Verification items for the finished model (mm, model axes). Face numbers are marked on the shaded views. A direction names the side the tool comes from. Round coordinates to 2 decimals unless told otherwise and drop trailing zeros. Loops run counter-clockwise (first coordinate to the right, second up) from the corner with the lowest first, then second, coordinate; pieces in that order, holes last. Notation, with made-up numbers: (52, 2.25) -> (78, 2.25) arc R30 ccw to (78, 30.25) -> close; hole circle Ø4 at (-28.75, 60.25). An arc over 180 degrees is marked (long way). Write item = value, one per line.
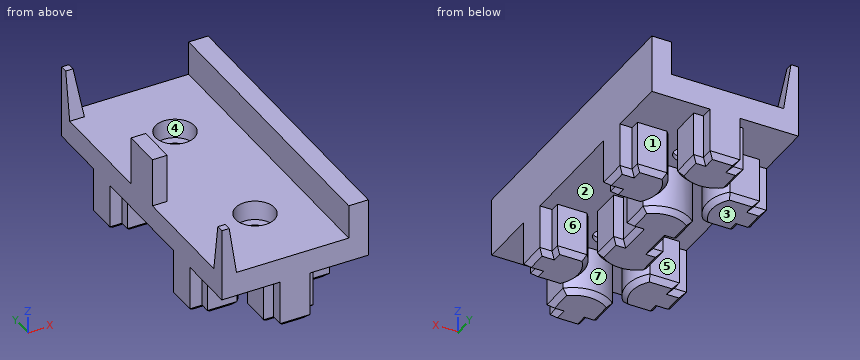
```python
from build123d import *

# Parameters (mm, degrees)
SKETCH_1_W                   = 30
SKETCH_1_H                   = 60
EXTRUDE_1_DEPTH              = 5
SKETCH_2_W                   = 3
SKETCH_2_H                   = 3
SKETCH_2_W_2                 = 4
SKETCH_2_H_2                 = 60
SKETCH_2_H_3                 = 8
EXTRUDE_2_DEPTH              = 10
CUT_EXTRUDE_1_DEPTH          = 44.058100283
CUT_EXTRUDE_3_DEPTH          = 7
SKETCH_5_W                   = 4
SKETCH_5_H                   = 3
CUT_EXTRUDE_4_DEPTH          = 64.639610307
HOLE_WIZARD_M4_1_D           = 4.5
HOLE_WIZARD_M4_1_CBORE_D     = 8
HOLE_WIZARD_M4_1_CBORE_DEPTH = 4
EXTRUDE_3_DEPTH              = 10
CHAMFER_1_SIZE               = 1


with BuildPart() as part:
    # 스케치1 → 보스-돌출1 (new body)
    with BuildSketch(Plane.XY):
        Rectangle(SKETCH_1_W, SKETCH_1_H)
    extrude(amount=EXTRUDE_1_DEPTH)

    # 스케치2 → 보스-돌출2 (add)
    with BuildSketch(Plane.XY.offset(5)):
        with Locations((-13.5, -28.5)):
            Rectangle(SKETCH_2_W, SKETCH_2_H)
        with Locations((-13.5, 28.5)):
            Rectangle(SKETCH_2_W, SKETCH_2_H)
        with Locations((13, 0)):
            Rectangle(SKETCH_2_W_2, SKETCH_2_H_2)
        with Locations((-13.5, 0)):
            Rectangle(SKETCH_2_W, SKETCH_2_H_3)
    extrude(amount=EXTRUDE_2_DEPTH)

    # 스케치3 → 컷-돌출1 (cut, through all)
    with BuildSketch(Plane(origin=(-12, 0, 0), x_dir=(0, 0, -1), z_dir=(1, 0, 0))):
        Polygon((-15, -28.5), (-5, -27), (-15, -27), align=None)
    cut_extrude_1 = extrude(amount=-CUT_EXTRUDE_1_DEPTH, mode=Mode.SUBTRACT)

    # 스케치4 → 컷-돌출3 (cut)
    with BuildSketch(Plane.XZ.offset(30)):
        Polygon((-13.5, 15), (-12, 15), (-12, 5), align=None)
    cut_extrude_3 = extrude(amount=-CUT_EXTRUDE_3_DEPTH, mode=Mode.SUBTRACT)

    # 대칭 복사1: 컷-돌출1, 컷-돌출3 across plane
    add(cut_extrude_1.mirror(Plane(origin=(0, 0, 0), x_dir=(0, 0, 1), z_dir=(0, -1, 0))), mode=Mode.SUBTRACT)
    add(cut_extrude_3.mirror(Plane(origin=(0, 0, 0), x_dir=(0, 0, 1), z_dir=(0, -1, 0))), mode=Mode.SUBTRACT)

    # 스케치5 → 컷-돌출4 (cut, through all)
    with BuildSketch(Plane(origin=(0, 30, 0), x_dir=(1, 0, 0), z_dir=(0, 1, 0))):
        with Locations((13, -13.5)):
            Rectangle(SKETCH_5_W, SKETCH_5_H)
    extrude(amount=-CUT_EXTRUDE_4_DEPTH, mode=Mode.SUBTRACT)

    # M4 소켓 머리 캡 나사용 카운터보어1 (through all)
    with Locations(Plane.XY.offset(5)):
        with Locations((0, -15), (0, 15)):
            CounterBoreHole(HOLE_WIZARD_M4_1_D / 2, HOLE_WIZARD_M4_1_CBORE_D / 2, HOLE_WIZARD_M4_1_CBORE_DEPTH)

    # 스케치9 → 보스-돌출3 (add)
    with BuildSketch(Plane(origin=(0, 0, 0), x_dir=(-1, 0, 0), z_dir=(0, 0, -1))):
        with BuildLine():
            Line((-3.05, 30), (3.05, 30))
            Line((3.05, 30), (3.05, 27.5))
            Line((3.05, 27.5), (5.05, 27.5))
            Line((5.05, 27.5), (5.05, 21.454957169))
            ThreePointArc((5.05, 21.454957169), (0, 19.5), (-5.05, 21.454957169))
            Line((-5.05, 21.454957169), (-5.05, 27.5))
            Line((-5.05, 27.5), (-3.05, 27.5))
            Line((-3.05, 27.5), (-3.05, 30))
        make_face()
        with BuildLine():
            Line((15, 18.05), (15, 11.95))
            Line((15, 11.95), (12.5, 11.95))
            Line((12.5, 11.95), (12.5, 9.95))
            Line((12.5, 9.95), (6.454957169, 9.95))
            ThreePointArc((6.454957169, 9.95), (4.5, 15), (6.454957169, 20.05))
            Line((6.454957169, 20.05), (12.5, 20.05))
            Line((12.5, 20.05), (12.5, 18.05))
            Line((12.5, 18.05), (15, 18.05))
        make_face()
        with BuildLine():
            Line((-3.05, 2.5), (-5.05, 2.5))
            Line((-5.05, 2.5), (-5.05, 8.545042831))
            ThreePointArc((-5.05, 8.545042831), (0, 10.5), (5.05, 8.545042831))
            Line((5.05, 8.545042831), (5.05, 2.5))
            Line((5.05, 2.5), (3.05, 2.5))
            Line((3.05, 2.5), (3.05, -2.5))
            Line((3.05, -2.5), (5.05, -2.5))
            Line((5.05, -2.5), (5.05, -8.545042831))
            ThreePointArc((5.05, -8.545042831), (0, -10.5), (-5.05, -8.545042831))
            Line((-5.05, -8.545042831), (-5.05, -2.5))
            Line((-5.05, -2.5), (-3.05, -2.5))
            Line((-3.05, -2.5), (-3.05, 2.5))
        make_face()
        with BuildLine():
            Line((-15, 11.95), (-15, 18.05))
            Line((-15, 18.05), (-12.5, 18.05))
            Line((-12.5, 18.05), (-12.5, 20.05))
            Line((-12.5, 20.05), (-6.454957169, 20.05))
            ThreePointArc((-6.454957169, 20.05), (-4.5, 15), (-6.454957169, 9.95))
            Line((-6.454957169, 9.95), (-12.5, 9.95))
            Line((-12.5, 9.95), (-12.5, 11.95))
            Line((-12.5, 11.95), (-15, 11.95))
        make_face()
        with BuildLine():
            Line((-5.05, -27.5), (-5.05, -21.454957169))
            ThreePointArc((-5.05, -21.454957169), (0, -19.5), (5.05, -21.454957169))
            Line((5.05, -21.454957169), (5.05, -27.5))
            Line((5.05, -27.5), (3.05, -27.5))
            Line((3.05, -27.5), (3.05, -30))
            Line((3.05, -30), (-3.05, -30))
            Line((-3.05, -30), (-3.05, -27.5))
            Line((-3.05, -27.5), (-5.05, -27.5))
        make_face()
        with BuildLine():
            Line((-12.5, -9.95), (-6.454957169, -9.95))
            ThreePointArc((-6.454957169, -9.95), (-4.5, -15), (-6.454957169, -20.05))
            Line((-6.454957169, -20.05), (-12.5, -20.05))
            Line((-12.5, -20.05), (-12.5, -18.05))
            Line((-12.5, -18.05), (-15, -18.05))
            Line((-15, -18.05), (-15, -11.95))
            Line((-15, -11.95), (-12.5, -11.95))
            Line((-12.5, -11.95), (-12.5, -9.95))
        make_face()
        with BuildLine():
            Line((12.5, -20.05), (6.454957169, -20.05))
            ThreePointArc((6.454957169, -20.05), (4.5, -15), (6.454957169, -9.95))
            Line((6.454957169, -9.95), (12.5, -9.95))
            Line((12.5, -9.95), (12.5, -11.95))
            Line((12.5, -11.95), (15, -11.95))
            Line((15, -11.95), (15, -18.05))
            Line((15, -18.05), (12.5, -18.05))
            Line((12.5, -18.05), (12.5, -20.05))
        make_face()
    extrude(amount=EXTRUDE_3_DEPTH)

    # 모따기1
    chamfer_1_edges = [part.edges().sort_by_distance(p)[0] for p in [
        (3.05, 28.75, -10),
        (4.05, 27.5, -10),
        (5.05, 24.477478584, -10),
        (0, 19.5, -10),
        (-5.05, 24.477478584, -10),
        (-4.05, 27.5, -10),
        (-3.05, 28.75, -10),
        (0, 30, -10),
        (-13.75, 18.05, -10),
        (-12.5, 19.05, -10),
        (-9.477478584, 20.05, -10),
        (-4.5, 15, -10),
        (-9.477478584, 9.95, -10),
        (-12.5, 10.95, -10),
        (-13.75, 11.95, -10),
        (-15, 15, -10),
        (3.05, 0, -10),
        (4.05, -2.5, -10),
        (5.05, -5.522521416, -10),
        (0, -10.5, -10),
        (-5.05, -5.522521416, -10),
        (-4.05, -2.5, -10),
        (-3.05, 0, -10),
        (-4.05, 2.5, -10),
        (-5.05, 5.522521416, -10),
        (0, 10.5, -10),
        (5.05, 5.522521416, -10),
        (4.05, 2.5, -10),
        (13.75, 11.95, -10),
        (12.5, 10.95, -10),
        (9.477478584, 9.95, -10),
        (4.5, 15, -10),
        (9.477478584, 20.05, -10),
        (12.5, 19.05, -10),
        (13.75, 18.05, -10),
        (15, 15, -10),
        (0, -19.5, -10),
        (5.05, -24.477478584, -10),
        (4.05, -27.5, -10),
        (3.05, -28.75, -10),
        (0, -30, -10),
        (-3.05, -28.75, -10),
        (-4.05, -27.5, -10),
        (-5.05, -24.477478584, -10),
        (4.5, -15, -10),
        (9.477478584, -9.95, -10),
        (12.5, -10.95, -10),
        (13.75, -11.95, -10),
        (15, -15, -10),
        (13.75, -18.05, -10),
        (12.5, -19.05, -10),
        (9.477478584, -20.05, -10),
        (-4.5, -15, -10),
        (-9.477478584, -20.05, -10),
        (-12.5, -19.05, -10),
        (-13.75, -18.05, -10),
        (-15, -15, -10),
        (-13.75, -11.95, -10),
        (-12.5, -10.95, -10),
        (-9.477478584, -9.95, -10),
    ]]
    chamfer(chamfer_1_edges, length=CHAMFER_1_SIZE)


solid = part.part
```
(1) Sectioned sample at B-B, the plane z = 8. Record the cut outline in (x, y), and give its area (3 significant figures).
Filled sheet:
outline = (-15, -30) -> (-12.45, -30) -> (-12.45, -27.45) -> (-15, -27.45) -> close; (-15, -4) -> (-12, -4) -> (-12, 4) -> (-15, 4) -> close; (-15, 27.45) -> (-12.45, 27.45) -> (-12.45, 30) -> (-15, 30) -> close; (11, -30) -> (15, -30) -> (15, 30) -> (11, 30) -> close
area = 277 mm2
(2) Go/stop test with flat-tipped pins: pin 1 Ø0.8 at (x, z) = (14, -4.5) entering from +Y; pin 2 Ø0.6 at (y, z) = (-18.5, -6) entering from -X; pin 3 Ø2 at (y, z) = (-28, -5.5) entering from -X; pin 4 Ø8 at (x, z) = (-5, -6) entering from +Y. Record where each tip stops, or that it passes through.
Filled sheet:
pin_1 = 18.05
pin_2 = -12.5
pin_3 = -5.05
pin_4 = 30
(3) Sectioned sample at A-A, the plane y = 15. Record the cut outline in (x, z), and give its area (4 significant figures).
Filled sheet:
outline = (-15, -9) -> (-14, -10) -> (-5.5, -10) -> (-4.5, -9) -> (-4.5, 0) -> (-2.25, 0) -> (-2.25, 1) -> (-4, 1) -> (-4, 5) -> (-15, 5) -> close; (2.25, 0) -> (4.5, 0) -> (4.5, -9) -> (5.5, -10) -> (14, -10) -> (15, -9) -> (15, 12) -> (11, 12) -> (11, 5) -> (4, 5) -> (4, 1) -> (2.25, 1) -> close
area = 349.5 mm2
(4) Set-up check for the marked faces 4, 5, 6 and 7: record each of +Z, -Z, +X, -X, +Y, -Y from which the full face is reachable in a straight line by a thin tool's end or side.
Filled sheet:
face_4 = +Z
face_5 = -Z, -X
face_6 = -Z, +X
face_7 = -Z
(5) Draft check along Y on the marked faces 1, 2 and 3. Enter one of: released by +Y, released by -Y, zero draft, split by the parting line, or undercut.
Filled sheet:
face_1 = released by +Y
face_2 = undercut
face_3 = zero draft
(6) Sectioned sample at C-C, the plane x = 0. Count the separate pieces of the cut face and the enclosed holes in it, and give its area (3 significant figures).
Filled sheet:
separate_pieces = 3
enclosed_holes = 0
area = 644 mm2
(7) Material ranges on probe 1 along Y at (x, z) = (0, 4.25); probe 2 along Y at (x, z) = (0, 0.75); probe 3 along Z at (x, y) = (4, -25), recorded low to high. Write a range as from..to.
Filled sheet:
probe_1 = -30..-19, -11..11, 19..30
probe_2 = -30..-17.25, -12.75..12.75, 17.25..30
probe_3 = -10..5
(8) Sectioned sample at D-D, the plane x = 10.25. Record the cut outline in (y, z).
Filled sheet:
outline = (-30, 0) -> (-20.05, 0) -> (-20.05, -9) -> (-19.05, -10) -> (-10.95, -10) -> (-9.95, -9) -> (-9.95, 0) -> (9.95, 0) -> (9.95, -9) -> (10.95, -10) -> (19.05, -10) -> (20.05, -9) -> (20.05, 0) -> (30, 0) -> (30, 5) -> (-30, 5) -> close
